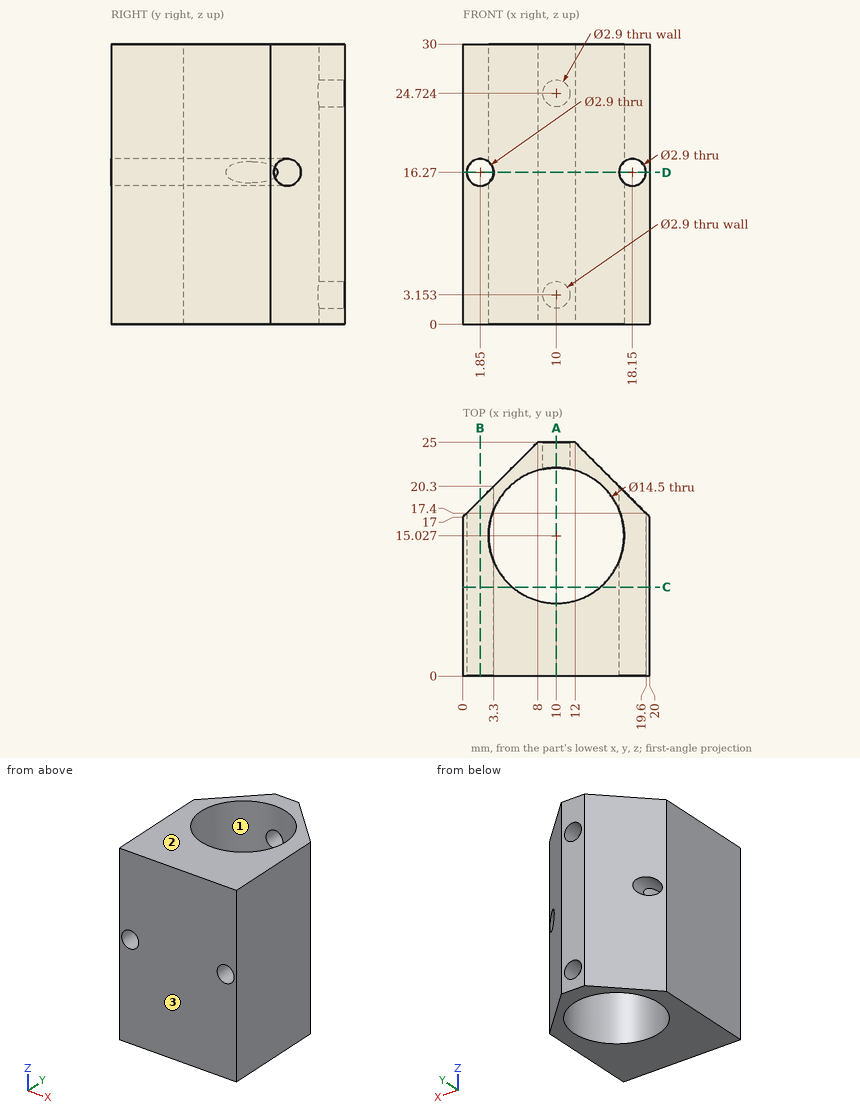
Geometry check sheet. Reference: drawing and pictorial views, mm from the part's lowest x, y, z. Round coordinates to 2 decimals unless told otherwise and drop trailing zeros. Loops run counter-clockwise (first coordinate to the right, second up) from the corner with the lowest first, then second, coordinate; pieces in that order, holes last. Notation, with made-up numbers: M -37,-38 L -5,-38 A17 cw -5,-15 Z; hole C 89.5,68.5 d2. An arc over 180 degrees is marked long. Return JSON: item names as keys, results as strings. Group by question number.
(1) Scan lines: line 1 along Z through (x, y) = (1.85, 14); line 2 along Z through (x, y) = (10, 23.85) (1 decimal); line 3 along Y through (x, z) = (10, 7.5). Record each from-to range of solid material in increasing order. Write a range as [from, to].
(2) Mould release check, pull along Y, two halves, no side actions. Record for the marked faces 1, 2 and 3: pulls with the +Y half, pulls with the -Y half, needs draft (parallel to the pull), parting line crosses it, or undercut.
(3) Section check B-B, the plane x = 1.85. Enter the section's corners in (y, z).
(4) Section check C-C, the plane y = 9.5. Enter the section's corners in (x, z), and give its area (3 significant figures).
(5) Go/stop test with flat-tipped pins: pin 1 (1 mm diameter, centred on y = 3.5, z = 19.5, fed in from -X); pin 2 (4 mm diameter, centred on x = 18.15, z = 16.27, fed in from +Y); pin 3 (1.7 mm diameter, centred on x = 1.85, z = 16.27, fed in from -Y); pin 4 (1.5 mm diameter, centred on x = 16.5, z = 5.5, fed in from +Y). Record where each tip stops, or that it passes through.
(6) Section check A-A, the plane x = 10. Enter the section's corners in (y, z) (1 decimal).
(7) Section check D-D, the plane z = 16.27. Enter the section's corners in (x, y).
Data:
{
 "1": {"line 1": "[0, 14.82], [17.72, 30]", "line 2": "[0, 1.7], [4.6, 23.3], [26.2, 30]", "line 3": "[0, 7.78], [22.28, 25]"},
 "2": {"face 1": "undercut", "face 2": "needs draft", "face 3": "pulls with the -Y half"},
 "3": {"outline": "M 0,0 L 18.85,0 L 18.85,14.82 L 0,14.82 Z; M 0,17.72 L 18.85,17.72 L 18.85,30 L 0,30 Z"},
 "4": {"outline": "M 0,0 L 5.31,0 L 5.31,30 L 0,30 Z; M 14.69,0 L 20,0 L 20,30 L 14.69,30 Z; hole C 1.85,16.27 d2.9; hole C 18.15,16.27 d2.9", "area": "305 mm²"},
 "5": {"pin 1": "x = 0", "pin 2": "y = 20.85", "pin 3": "through", "pin 4": "y = 21.25"},
 "6": {"outline": "M 0,0 L 7.8,0 L 7.8,30 L 0,30 Z; M 22.3,0 L 25,0 L 25,1.7 L 22.3,1.7 Z; M 22.3,4.6 L 25,4.6 L 25,23.3 L 22.3,23.3 Z; M 22.3,26.2 L 25,26.2 L 25,30 L 22.3,30 Z"},
 "7": {"outline": "M 0,0 L 0.4,0 L 0.4,17.4 L 0,17 Z; M 3.3,0 L 16.7,0 L 16.7,12.26 A7.25 cw 3.3,12.26 Z; M 3.3,17.8 A7.25 cw 16.7,17.8 L 16.7,20.3 L 12,25 L 8,25 L 3.3,20.3 Z; M 19.6,0 L 20,0 L 20,17 L 19.6,17.4 Z"}
}
